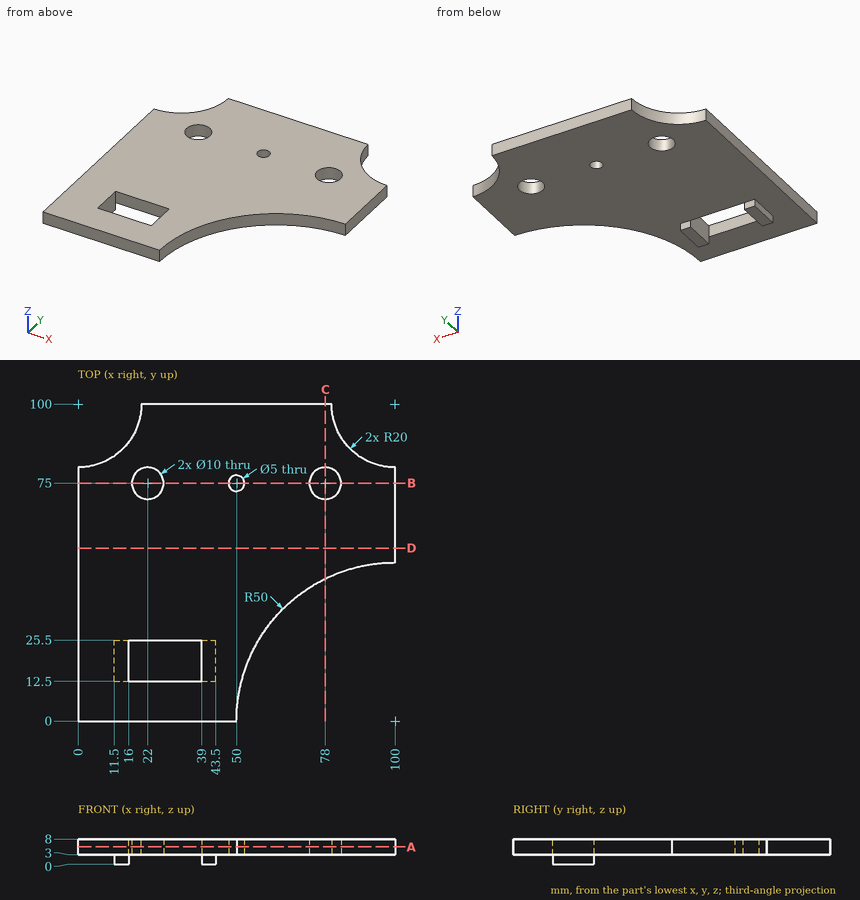
The figure shows three views and two pictorial views of one solid part (mm, origin at its lowest corner). Answer the questions. Give positions to 0.01 mm unless a question says otherwise; leave off trailing zeros. Write each loop counter-clockwise with the first axis right and the second up, starting at its lowest first coordinate (ties: lowest second). Pieces come first, ordered by that corner, then holes. Notation, with made-up numbers: M -8.5,41.25 L 19.5,41.25 A24 cw 19.5,76.25 Z; hole C -32,7 d6. An arc over 180 degrees is marked long. One line per item, written item: value. Start each with the question number.
(1) Find the intervals of material crossed by line 1 (Y direction, x = 22, z = 7); line 2 (Y direction, x = 31, z = 5.5); line 3 (X direction, y = 25, z = 1.75), in increasing order.
(2) Flat-ended cylindrical pins translate along their axes: pin 1 Ø1.5 at (y, z) = (19, 1) entering from +X; pin 2 Ø1.5 at (y, z) = (87, 1.5) entering from +X; pin 3 Ø3.5 at (x, z) = (41, 2) entering from -Y; pin 4 Ø0.9 at (x, z) = (13, 1.5) entering from +Y. Find the tip coordinate at first contact, or state that the pin passes through.
(3) Find section A-A (z = 5.5). Determine the outline of the cut face in (x, y).
(4) Find section D-D (y = 54.5). Determine the outline of the cut face in (x, z).
(5) Find section C-C (x = 78). Determine the outline of the cut face in (y, z).
(6) Find section B-B (y = 75). Determine the outline of the cut face in (x, z).
Results below:
1. line 1: y = 0 to 12.5, 25.5 to 70, 80 to 100
1. line 2: y = 0 to 12.5, 25.5 to 100
1. line 3: x = 11.5 to 16, 39 to 43.5
2. pin 1: stops at x = 43.5
2. pin 2: passes through
2. pin 3: stops at y = 0
2. pin 4: stops at y = 25.5
3. outline: M 0,0 L 50,0 A50 cw 100,50 L 100,80 A20 cw 80,100 L 20,100 A20 cw 0,80 Z; hole M 16,12.5 L 39,12.5 L 39,25.5 L 16,25.5 Z; hole C 22,75 d10; hole C 50,75 d5; hole C 78,75 d10
4. outline: M 0,3 L 100,3 L 100,8 L 0,8 Z
5. outline: M 44.9,3 L 70,3 L 70,8 L 44.9,8 Z; M 80,3 L 100,3 L 100,8 L 80,8 Z
6. outline: M 0,3 L 17,3 L 17,8 L 0,8 Z; M 27,3 L 47.5,3 L 47.5,8 L 27,8 Z; M 52.5,3 L 73,3 L 73,8 L 52.5,8 Z; M 83,3 L 100,3 L 100,8 L 83,8 Z
